from build123d import *

# Parameters (mm, degrees)
EXTRUSION1_DEPTH = 50
EXTRUSION2_REACH = 17.556
ESQUISSE3_R      = 2.5
EXTRUSION3_REACH = 27.142
ESQUISSE4_R      = 1.5


with BuildPart() as part:
    # Esquisse1 → Extrusion1 (new body)
    with BuildSketch(Plane(origin=(0, 0, 0), x_dir=(1, 0, 0), z_dir=(0, 1, 0))):
        Polygon((0, 0), (0, 20), (14.142135624, 34.142135624), (15.556349186, 32.727922061), (2, 19.171572875), (2, 0), align=None)
    extrude(amount=EXTRUSION1_DEPTH)

    # Esquisse3 → Extrusion2 (cut, up to next)
    with BuildSketch(Plane.ZY, mode=Mode.PRIVATE) as extrusion2_sk1:
        with Locations((-10, 5)):
            Circle(ESQUISSE3_R)
    extrusion2_tool1 = extrude(extrusion2_sk1.sketch, amount=-EXTRUSION2_REACH, mode=Mode.PRIVATE) & part.part
    add(extrusion2_tool1.solids().sort_by_distance((0, 5, -10))[0], mode=Mode.SUBTRACT)
    # Esquisse3 → Extrusion2 (cut, up to next)
    with BuildSketch(Plane.ZY, mode=Mode.PRIVATE) as extrusion2_sk2:
        with Locations((-10, 45)):
            Circle(ESQUISSE3_R)
    extrusion2_tool2 = extrude(extrusion2_sk2.sketch, amount=-EXTRUSION2_REACH, mode=Mode.PRIVATE) & part.part
    add(extrusion2_tool2.solids().sort_by_distance((0, 45, -10))[0], mode=Mode.SUBTRACT)

    # Esquisse4 → Extrusion3 (cut, up to next)
    with BuildSketch(Plane(origin=(-10, 0, -10), x_dir=(-0.707106781, 0, 0.707106781), z_dir=(-0.707106781, 0, -0.707106781)), mode=Mode.PRIVATE) as extrusion3_sk1:
        with Locations((-24.142135624, 46)):
            Circle(ESQUISSE4_R)
    extrusion3_tool1 = extrude(extrusion3_sk1.sketch, amount=-EXTRUSION3_REACH, mode=Mode.PRIVATE) & part.part
    add(extrusion3_tool1.solids().sort_by_distance((7.071068, 46, -27.071068))[0], mode=Mode.SUBTRACT)
    # Esquisse4 → Extrusion3 (cut, up to next)
    with BuildSketch(Plane(origin=(-10, 0, -10), x_dir=(-0.707106781, 0, 0.707106781), z_dir=(-0.707106781, 0, -0.707106781)), mode=Mode.PRIVATE) as extrusion3_sk2:
        with Locations((-24.142135624, 4)):
            Circle(ESQUISSE4_R)
    extrusion3_tool2 = extrude(extrusion3_sk2.sketch, amount=-EXTRUSION3_REACH, mode=Mode.PRIVATE) & part.part
    add(extrusion3_tool2.solids().sort_by_distance((7.071068, 4, -27.071068))[0], mode=Mode.SUBTRACT)


solid = part.part
Work out the finished part from the listing and answer in its coordinate system (mm). A direction names the side the tool comes from. Round coordinates to 2 decimals unless told otherwise and drop trailing zeros. Order: outer loops, then holes, each group sorted by start corner. A loop starts at its lowest first (then second) coordinate and runs counter-clockwise, first axis right, second up. Notation, with made-up numbers: M 68,48 L 127,48 A25 cw 127,61 Z; hole C -19,4 d11. An arc over 180 degrees is marked long. Put each result on its own line as item: value. Start each with the question number.
Q1. Straight lines are drawn through the part: L1, parallel to Y at x = 0.4, z = -10; L2, parallel to X at y = 15.5, z = -10.5; L3, parallel to Z at x = 4.25, y = 8. For each, find the intervals that lie inside material, in ascending order. Write a range as [from, to].
Q2. Section A-A, the plane z = -10 is taken. Write down the section's boundary in (x, y).
Q3. Section C-C, the plane y = 16 is taken. Write down the section's boundary in (x, z).
Q4. For a pull along X with two mould halves and no side action, classify faces 3 (the flat face through (0, 25, -10)), 4 (the cylindrical face through (0.99, 42.56, -10.54)), 5 (the cylindrical face through (6.76, 4.45, -25.36)) as pulls with the +X half, pulls with the -X half, needs draft (parallel to the pull), parting line crosses it, or undercut.
Q5. Flat-ended cylindrical pins translate along their axes: pin 1 (10 mm diameter, centred on y = 24.5, z = -3.5, fed in from +X); pin 2 (3 mm diameter, centred on x = 7.5, y = 43.5, fed in from +Z); pin 3 (3 mm diameter, centred on y = 5, z = -10, fed in from -X); pin 4 (5 mm diameter, centred on x = 12.5, y = 32.5, fed in from -Z). Find the tip coordinate at first contact, or state that the pin passes through.
Q6. Section B-B, the plane x = 1.25 is taken. Write down the section's boundary in (y, z), and give its area (3 significant figures).
Q7. A tool of negligible diameter and unlimited length cuts with its end or side. For faces 1 (the flat face through (2, 25, -10)), 2 (the flat face through (3, 50, -21)), from which of +Z, -Z, +X, -X, +Y, -Y can it reach the whole face along a straight path? Write none if from no direction.
Q8. Section D-D, the plane z = -3 is taken. Write down the section's boundary in (x, y).
Findings below:
1. L1: y = [0, 2.5], [7.5, 42.5], [47.5, 50]
1. L2: x = [0, 2]
1. L3: z = [-24.25, -21.42]
2. outline: M 0,0 L 2,0 L 2,2.5 L 0,2.5 Z; M 0,7.5 L 2,7.5 L 2,42.5 L 0,42.5 Z; M 0,47.5 L 2,47.5 L 2,50 L 0,50 Z
3. outline: M 0,-20 L 14.14,-34.14 L 15.56,-32.73 L 2,-19.17 L 2,0 L 0,0 Z
4. face 3: pulls with the -X half
4. face 4: needs draft
4. face 5: undercut
5. pin 1: stops at x = 2
5. pin 2: stops at z = -23.17
5. pin 3: passes through
5. pin 4: stops at z = -34.14
6. outline: M 0,-21.25 L 50,-21.25 L 50,0 L 0,0 Z; hole C 5,-10 d5; hole C 45,-10 d5
6. area: 1,020 mm^2
7. face 1: +Z, +X, +Y, -Y
7. face 2: +Z, -Z, +X, -X, +Y
8. outline: M 0,0 L 2,0 L 2,50 L 0,50 Z
